Geometry: see drawing. Coordinates: mm, zero at the bounding-box minimum. A direction names the side the tool comes from. Coordinates: 2 decimals unless noted, no trailing zeros. Loops run counter-clockwise (first coordinate to the right, second up) from the corner with the lowest first, then second, coordinate; pieces in that order, holes last. Notation, with made-up numbers: (59, 47.5) -> (84, 47.5) arc R15 ccw to (84, 55.5) -> close; hole circle Ø8 at (89, 14.5). An arc over 180 degrees is marked (long way). Put each result on its own line as item: value. Start each with the question number.
1) Set-up query: the marked faces 3, 4 and 5. Return all of +Z, -Z, +X, -X, +Y, -Y with unobstructed straight access to the full face (end or side cutting, diameter ignored); none if empty.
2) Cut plane C-C (y = 12.5). Return the cut outline in (x, z).
3) Cut plane A-A (x = 25). Return the cut outline in (y, z).
4) Cut plane B-B (z = 10.5). Return the cut outline in (x, y).
5) Cut plane D-D (x = 15). Return the cut outline in (y, z), plus the area to 3 significant figures.
6) Contact query for flat-ended pins moving along their axis: P1, Ø8, axis at x = 22.5, y = 27, coming from the +Z side; P2, Ø5, axis at x = 6.5, y = 18, coming from the +Z side; P3, Ø1.2, axis at x = 5, y = 16.5, coming from the +Z side. Output: stop coordinate, or through.
7) Material intervals for L1, parallel to Z at x = 15, y = 6.25; L2, parallel to Y at x = 14.5, z = 22.5; L3, parallel to Z at x = 15, y = 17, sorted ascending.
8) Pull-direction query (Z, two-part tool) for the marked faces 1 and 2; classes: pulls with the +Z half, pulls with the -Z half, needs draft (parallel to the pull), parting line crosses it, or undercut.
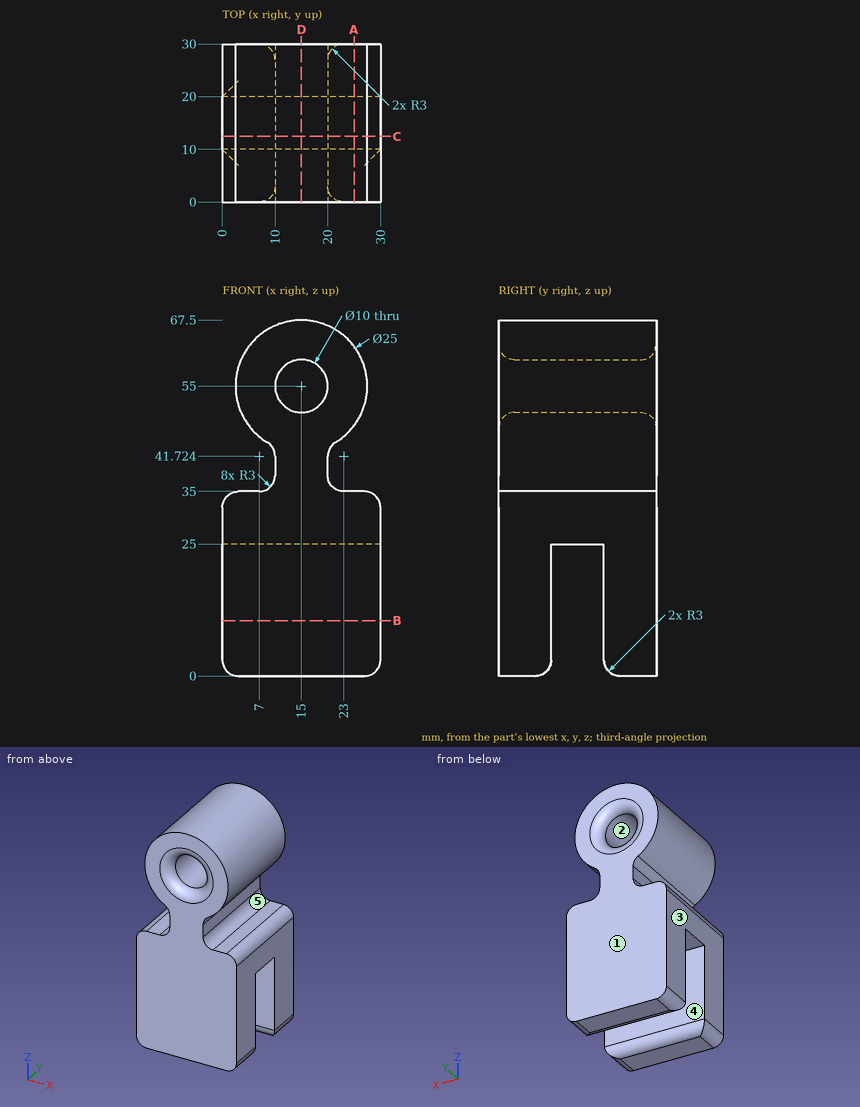
Results found:
1. face 3: +Z, -Z, -X, +Y, -Y
1. face 4: -Z, +X, -X
1. face 5: +X, +Y, -Y
2. outline: (0, 25) -> (30, 25) -> (30, 32) arc R3 ccw to (27, 35) -> (23, 35) arc R3 cw to (20, 38) -> (20, 41.72) arc R3 cw to (21.45, 44.29) arc R12.5 ccw (long way) to (8.55, 44.29) arc R3 cw to (10, 41.72) -> (10, 38) arc R3 cw to (7, 35) -> (3, 35) arc R3 ccw to (0, 32) -> close; hole circle Ø10 at (15, 55)
3. outline: (0, 0) -> (7, 0) arc R3 ccw to (10, 3) -> (10, 25) -> (20, 25) -> (20, 3) arc R3 ccw to (23, 0) -> (30, 0) -> (30, 35) -> (0, 35) -> close; (0, 47.5) -> (30, 47.5) -> (30, 62.5) -> (0, 62.5) -> close
4. outline: (0, 0) -> (30, 0) -> (30, 10) -> (0, 10) -> close; (0, 20) -> (30, 20) -> (30, 30) -> (0, 30) -> close
5. outline: (0, 0) -> (7, 0) arc R3 ccw to (10, 3) -> (10, 25) -> (20, 25) -> (20, 3) arc R3 ccw to (23, 0) -> (30, 0) -> (30, 47) arc R3 ccw to (27, 50) -> (3, 50) arc R3 ccw to (0, 47) -> close; (0, 63) arc R3 ccw to (3, 60) -> (27, 60) arc R3 ccw to (30, 63) -> (30, 67.5) -> (0, 67.5) -> close
5. area: 1,460 mm2
6. P1: stops at z = 67
6. P2: stops at z = 65.97
6. P3: stops at z = 63.24
7. L1: z = 0 to 50, 60 to 67.5
7. L2: y = 0 to 10, 20 to 30
7. L3: z = 25 to 50, 60 to 67.5
8. face 1: needs draft
8. face 2: undercut
